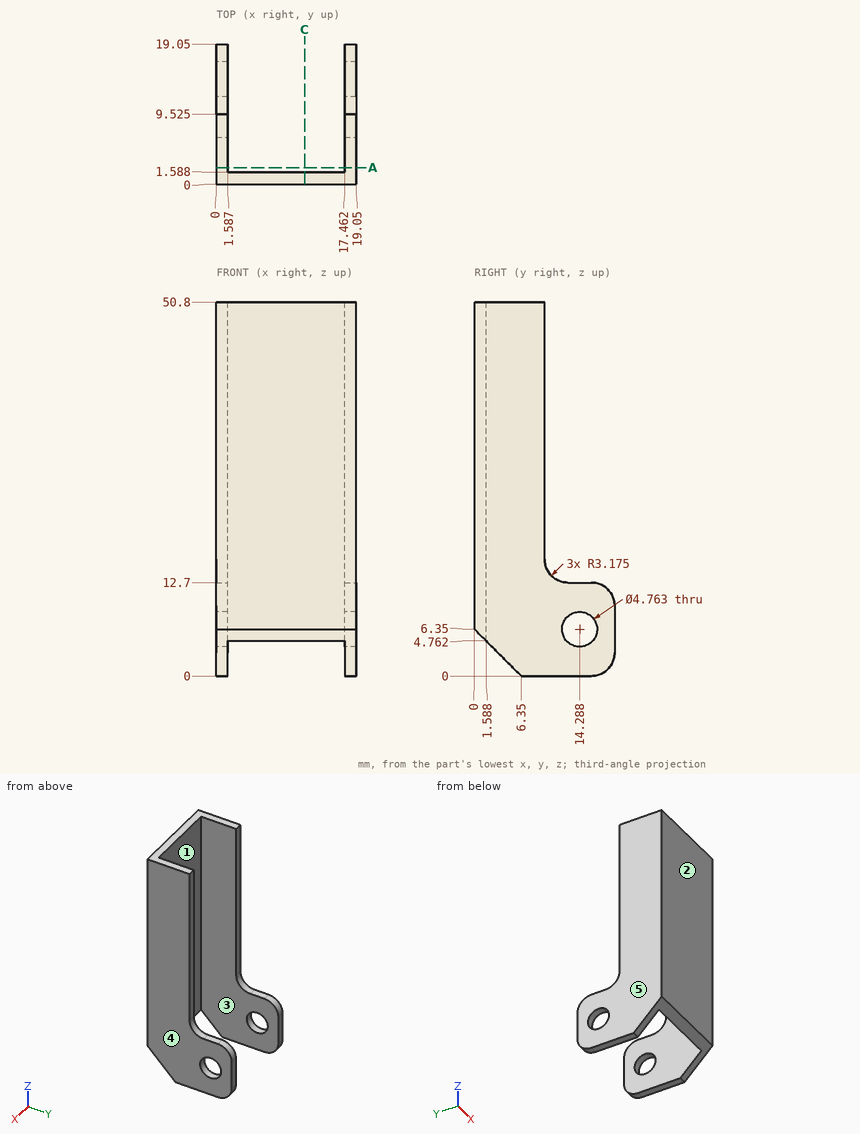
Answer from the drawing. Dimensions are ordinates in mm from the lowest x, y and z of the part. A direction names the side the tool comes from. Give positions to 0.01 mm unless a question says otherwise; leave off trailing zeros. Loops run counter-clockwise (first coordinate to the right, second up) from the corner with the lowest first, then second, coordinate; pieces in that order, holes last. Notation, with made-up numbers: (-29, 61) -> (-4, 61) arc R12 ccw to (-4, 71) -> close; hole circle Ø11 at (24, -21). An arc over 180 degrees is marked (long way). Use a Markdown table: item, result.
Q1. Section C-C, the plane x = 12 is taken. Determine the outline of the cut face in (y, z).
Solved:
| item | result |
|---|---|
| outline | (0, 6.35) -> (1.59, 4.76) -> (1.59, 50.8) -> (0, 50.8) -> close |
Q2. A tool of negligible diameter and unlimited length cuts with its end or side. For the marked faces 1 and 2, from which of +Z, -Z, +X, -X, +Y, -Y can it reach the whole face along a straight path? Write none if from no direction.
Solved:
| item | result |
|---|---|
| face 1 | +Z, -Z, +Y |
| face 2 | +Z, -Z, +X, -X, -Y |
Q3. Each of these flat-tipped pins is pushed along its axis until it touches: pin 1 (1.3 mm diameter, centred on x = 18, z = 32.5, fed in from +Y) (1 decimal); pin 2 (5 mm diameter, centred on y = 7.5, z = 30.5, fed in from -X); pin 3 (1.3 mm diameter, centred on x = 0.5, y = 15, fed in from +Z); pin 4 (5 mm diameter, centred on y = 14, z = 23.5, fed in from +X). Where does it stop, or does it pass through?
Solved:
| item | result |
|---|---|
| pin 1 | stops at y = 9.5 |
| pin 2 | stops at x = 0 |
| pin 3 | stops at z = 12.7 |
| pin 4 | passes through |
Q4. Find the intervals of material crossed by line 1 along Z through (x, y) = (17.75, 14.25); line 2 along X through (y, z) = (10.5, 11.5); line 3 along Y through (x, z) = (2, 48), in increasing order.
Solved:
| item | result |
|---|---|
| line 1 | z = 0 to 3.97, 8.73 to 12.7 |
| line 2 | x = 0 to 1.59, 17.46 to 19.05 |
| line 3 | y = 0 to 1.59 |
Q5. Section A-A, the plane y = 2.25 is taken. Determine the outline of the cut face in (x, z), then the cut area to 3 significant figures.
Solved:
| item | result |
|---|---|
| outline | (0, 4.1) -> (1.59, 4.1) -> (1.59, 50.8) -> (0, 50.8) -> close; (17.46, 4.1) -> (19.05, 4.1) -> (19.05, 50.8) -> (17.46, 50.8) -> close |
| area | 148 mm^2 |
Q6. Determine the mould class of the marked faces 3, 4 and 5 for opening direction X: pulls with the +X half, pulls with the -X half, needs draft (parallel to the pull), parting line crosses it, or undercut.
Solved:
| item | result |
|---|---|
| face 3 | undercut |
| face 4 | pulls with the +X half |
| face 5 | pulls with the -X half |
